Build history of the part. All positions in model axes, mm. Face numbers are marked on the shaded views. A direction names the side the tool comes from. Give positions to 0.01 mm unless a question says otherwise; leave off trailing zeros. Write each loop counter-clockwise with the first axis right and the second up, starting at its lowest first coordinate (ties: lowest second). Pieces come first, ordered by that corner, then holes. Notation, with made-up numbers: M 28.25,-34.75 L 45.25,-34.75 A17 cw 45.25,-5.75 Z; hole C 77,-33 d10. An arc over 180 degrees is marked long. Return JSON: item names as keys, results as strings. Group by question number.
Q1. Wall check: probe 1 along X at (y, z) = (6.25, 0); probe 2 along X at (y, z) = (10.5, -15.5). Give the ranges that are in metal, low to high.
Q2. Pull direction X, two halves, no side cores. Call the marked faces 1, 2 and 3: +X half, -X half, draft (parallel to the pull), parting line (faces both ways), or undercut.
Q3. Tool access for the marked faces 4, 5 and 6: list every direction of +Z, -Z, +X, -X, +Y, -Y with a clear straight run to the whole face (end or side of a thin tool).
Q4. Band-saw the part on C-C, the plane x = 13.97. Give the cut face in (y, z) (3 decimals).
Q5. Band-saw the part on B-B, the plane z = 0. Give the cut face in (x, y) (1 decimal).
Q6. Flat gauge pins, fed straight in: pin 1 Ø2 at (y, z) = (9.5, -17) entering from -X; pin 2 Ø3.5 at (x, z) = (13, -13.5) entering from -Y; pin 3 Ø1 at (y, z) = (6, 3) entering from +X. Where does each tip first touch, or does it go through?
Q7. Band-saw the part on D-D, the plane x = 7. Give the cut face in (y, z) (3 decimals), then the cut area to 3 significant figures.
Q8. Band-saw the part on A-A, the plane y = 1.25. Give the cut face in (x, z), then the cut area to 3 significant figures.
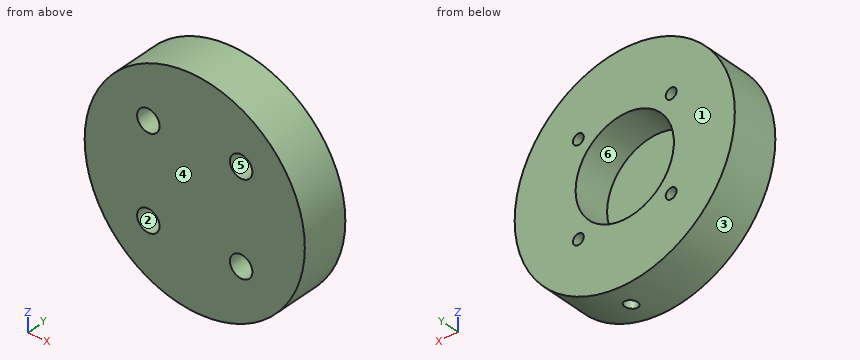
from build123d import *

# Parameters (mm, degrees)
SKETCH2_R                                           = 33.147
BOSS_EXTRUDE1_DEPTH                                 = 14.224
SKETCH4_R                                           = 14.7955
CUT_EXTRUDE1_DEPTH                                  = 11.049
F_24_0_152_DIAMETER_HOLE1_D                         = 3.8608
F_24_0_152_DIAMETER_HOLE1_DEPTH                     = 25.4
F_24_0_152_DIAMETER_HOLE1_TIP                       = 1.159901339
F_24_0_152_DIAMETER_HOLE1_ON_FACE_2_D               = 3.8608
F_24_0_152_DIAMETER_HOLE1_ON_FACE_2_DEPTH           = 25.4
F_24_0_152_DIAMETER_HOLE1_ON_FACE_2_TIP             = 1.159901339
CBORE_FOR_4_BINDING_HEAD_MACHINE_SCREW1_D           = 3.2639
CBORE_FOR_4_BINDING_HEAD_MACHINE_SCREW1_CBORE_D     = 6.74624
CBORE_FOR_4_BINDING_HEAD_MACHINE_SCREW1_CBORE_DEPTH = 11.049


with BuildPart() as part:
    # Sketch2 → Boss-Extrude1 (new body)
    with BuildSketch(Plane(origin=(0, 0, 0), x_dir=(1, 0, 0), z_dir=(0, 1, 0))):
        Circle(SKETCH2_R)
    extrude(amount=BOSS_EXTRUDE1_DEPTH)

    # Sketch4 → Cut-Extrude1 (cut)
    with BuildSketch(Plane(origin=(0, 14.224, 0), x_dir=(1, 0, 0), z_dir=(0, 1, 0))):
        Circle(SKETCH4_R)
    extrude(amount=-CUT_EXTRUDE1_DEPTH, mode=Mode.SUBTRACT)

    # #24 (0.152) Diameter Hole1
    with Locations(Plane(origin=(4.199730969, 7.112, -32.879870267), x_dir=(-0.991941059, 0, -0.126700183), z_dir=(0.126700183, 0, -0.991941059))):
        with Locations((0, 0)):
            Hole(F_24_0_152_DIAMETER_HOLE1_D / 2, depth=F_24_0_152_DIAMETER_HOLE1_DEPTH)
            with Locations((0, 0, -(F_24_0_152_DIAMETER_HOLE1_DEPTH + F_24_0_152_DIAMETER_HOLE1_TIP / 2))):  # 118° drill point
                Cone(0, F_24_0_152_DIAMETER_HOLE1_D / 2, F_24_0_152_DIAMETER_HOLE1_TIP, mode=Mode.SUBTRACT)

    # #24 (0.152) Diameter Hole1 on face 2
    with Locations(Plane(origin=(55.026579736, -11.282884423, 0), x_dir=(-0.991941059, 0, -0.126700183), z_dir=(0.126700183, 0, -0.991941059))):
        with Locations((0, 0)):
            Hole(F_24_0_152_DIAMETER_HOLE1_ON_FACE_2_D / 2, depth=F_24_0_152_DIAMETER_HOLE1_ON_FACE_2_DEPTH)
            with Locations((0, 0, -(F_24_0_152_DIAMETER_HOLE1_ON_FACE_2_DEPTH + F_24_0_152_DIAMETER_HOLE1_ON_FACE_2_TIP / 2))):  # 118° drill point
                Cone(0, F_24_0_152_DIAMETER_HOLE1_ON_FACE_2_D / 2, F_24_0_152_DIAMETER_HOLE1_ON_FACE_2_TIP, mode=Mode.SUBTRACT)

    # CBORE for #4 Binding Head Machine Screw1 (through all)
    with Locations(Plane(origin=(0, 0, 0), x_dir=(-1, 0, 0), z_dir=(0, -1, 0))):
        with Locations((13.97, -13.97), (-13.97, -13.97), (-13.97, 13.97), (13.97, 13.97)):
            CounterBoreHole(CBORE_FOR_4_BINDING_HEAD_MACHINE_SCREW1_D / 2, CBORE_FOR_4_BINDING_HEAD_MACHINE_SCREW1_CBORE_D / 2, CBORE_FOR_4_BINDING_HEAD_MACHINE_SCREW1_CBORE_DEPTH)


solid = part.part
From the geometry:
{
 "1": {"probe 1": "x = -33.15 to -14.8, 14.8 to 33.15", "probe 2": "x = -29.3 to -16.98, -10.96 to 10.96, 16.98 to 29.3"},
 "2": {"face 1": "draft", "face 2": "undercut", "face 3": "parting line"},
 "3": {"face 4": "+Z, -Z, +X, -X, -Y", "face 5": "-Y", "face 6": "+Y"},
 "4": {"outline": "M 0,-30.059 L 14.224,-30.059 L 14.224,-15.602 L 11.049,-15.602 L 11.049,-17.343 L 0,-17.343 Z; M 0,-10.597 L 11.049,-10.597 L 11.049,-12.338 L 14.224,-12.338 L 14.224,-4.873 L 3.175,-4.873 L 3.175,4.873 L 14.224,4.873 L 14.224,12.338 L 11.049,12.338 L 11.049,10.597 L 0,10.597 Z; M 0,17.343 L 11.049,17.343 L 11.049,15.602 L 14.224,15.602 L 14.224,30.059 L 0,30.059 Z"},
 "5": {"outline": "M -33.1,0 L 33.1,0 L 33.1,14.2 L 14.8,14.2 L 14.8,3.2 L -14.8,3.2 L -14.8,14.2 L -33.1,14.2 Z"},
 "6": {"pin 1": "stops at x = -29.03", "pin 2": "stops at y = 11.05", "pin 3": "stops at x = 33.05"},
 "7": {"outline": "M 0,-32.399 L 14.224,-32.399 L 14.224,-13.035 L 3.175,-13.035 L 3.175,13.035 L 14.224,13.035 L 14.224,32.399 L 0,32.399 Z", "area": "634 mm^2"},
 "8": {"outline": "C 0,0 d66.29; hole C -13.97,-13.97 d6.75; hole C -13.97,13.97 d6.75; hole C 13.97,-13.97 d6.75; hole C 13.97,13.97 d6.75", "area": "3,310 mm^2"}
}
